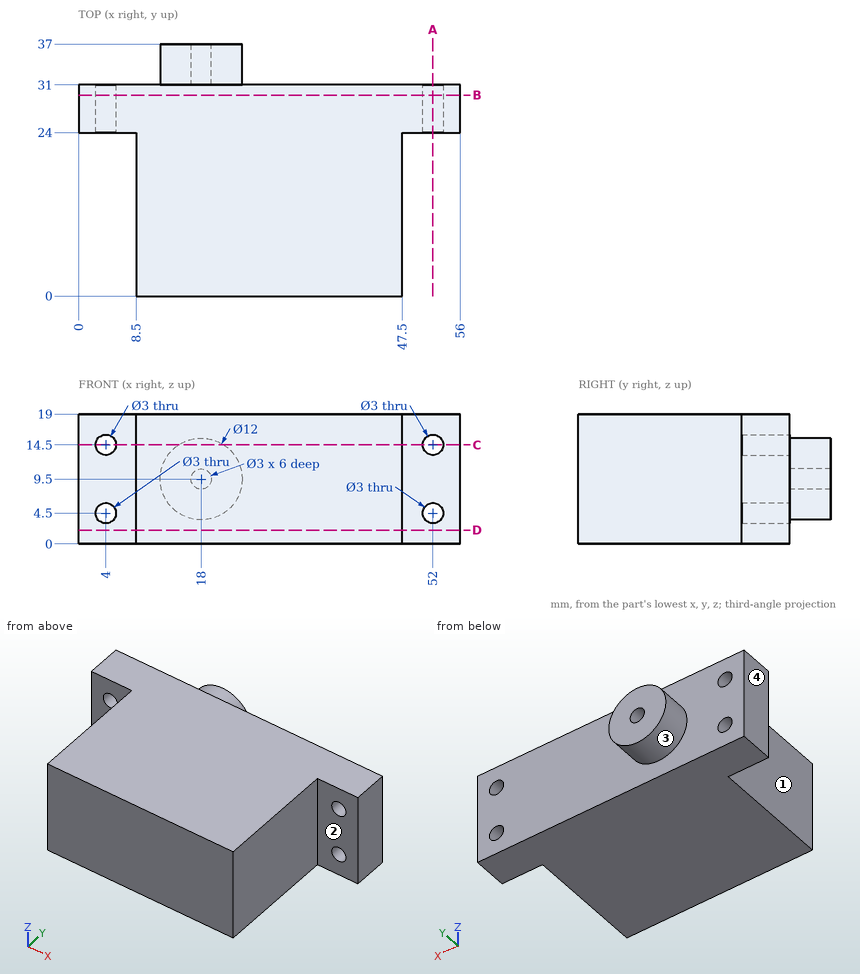
Part print with two shaded views. Sizes in mm from the minimum x, y, z corner. A direction names the side the tool comes from. Round coordinates to 2 decimals unless told otherwise and drop trailing zeros. Loops run counter-clockwise (first coordinate to the right, second up) from the corner with the lowest first, then second, coordinate; pieces in that order, holes last. Notation, with made-up numbers: (32.25, -38) - (72.25, -38) arc R21 ccw to (72.25, -6) - close; hole circle Ø8 at (5.5, 62.25). An arc over 180 degrees is marked (long way). Answer as a JSON object with one key per item and string values.
Item 1: Band-saw the part on C-C on z = 14.5. List the corners of the cut face in (x, y), plus the area to 3 significant figures.
Output:
{"outline": "(0, 24) - (2.5, 24) - (2.5, 31) - (0, 31) - close; (5.5, 24) - (8.5, 24) - (8.5, 0) - (47.5, 0) - (47.5, 24) - (50.5, 24) - (50.5, 31) - (21.32, 31) - (21.32, 37) - (14.68, 37) - (14.68, 31) - (5.5, 31) - close; (53.5, 24) - (56, 24) - (56, 31) - (53.5, 31) - close", "area": "1,330 mm2"}
Item 2: Pin check, flat tips, straight feed: pin 1 (4 mm diameter, centred on x = 4, z = 4.5, fed in from -Y); pin 2 (2.5 mm diameter, centred on x = 52, z = 4.5, fed in from +Y); pin 3 (5 mm diameter, centred on x = 6.5, z = 15.5, fed in from +Y). Stop position of each tip, or through.
Output:
{"pin 1": "y = 24", "pin 2": "through", "pin 3": "y = 31"}
Item 3: Band-saw the part on D-D on z = 2. List the corners of the cut face in (x, y).
Output:
{"outline": "(0, 24) - (8.5, 24) - (8.5, 0) - (47.5, 0) - (47.5, 24) - (56, 24) - (56, 31) - (0, 31) - close"}
Item 4: Band-saw the part on A-A on x = 52. List the corners of the cut face in (y, z).
Output:
{"outline": "(24, 0) - (31, 0) - (31, 3) - (24, 3) - close; (24, 6) - (31, 6) - (31, 13) - (24, 13) - close; (24, 16) - (31, 16) - (31, 19) - (24, 19) - close"}
Item 5: Wall check: L1, parallel to Z at x = 4, y = 27; L2, parallel to X at y = 27.25, z = 14.5; L3, parallel to X at y = 35.25, z = 9.5. Give the ranges that are in metal, low to high.
Output:
{"L1": "0 to 3, 6 to 13, 16 to 19", "L2": "0 to 2.5, 5.5 to 50.5, 53.5 to 56", "L3": "12 to 16.5, 19.5 to 24"}
Item 6: Band-saw the part on B-B on y = 29.5. List the corners of the cut face in (x, z), plus the area to 3 significant figures.
Output:
{"outline": "(0, 0) - (56, 0) - (56, 19) - (0, 19) - close; hole circle Ø3 at (4, 4.5); hole circle Ø3 at (4, 14.5); hole circle Ø3 at (52, 4.5); hole circle Ø3 at (52, 14.5)", "area": "1,040 mm2"}
Item 7: Tool access for the marked faces 1, 2, 3 and 4: list every direction of +Z, -Z, +X, -X, +Y, -Y with a clear straight run to the whole face (end or side of a thin tool).
Output:
{"face 1": "+Z, -Z, -X, -Y", "face 2": "+Z, -Z, +X, -Y", "face 3": "+Y", "face 4": "+Z, -Z, -X, +Y, -Y"}
